For this review, use the dimensioned drawing (mm, ordinates from the lowest corner) and the shaded views. A direction names the side the tool comes from. Coordinates: 2 decimals unless noted, no trailing zeros. Write each loop counter-clockwise with the first axis right and the second up, starting at its lowest first coordinate (ties: lowest second). Pieces come first, ordered by that corner, then holes. Notation, with made-up numbers: (30, -12.75) - (88, -12.75) arc R30 cw to (88, 18.25) - close; hole circle Ø3 at (86.25, 82). An arc over 180 degrees is marked (long way). One line per item, written item: value.
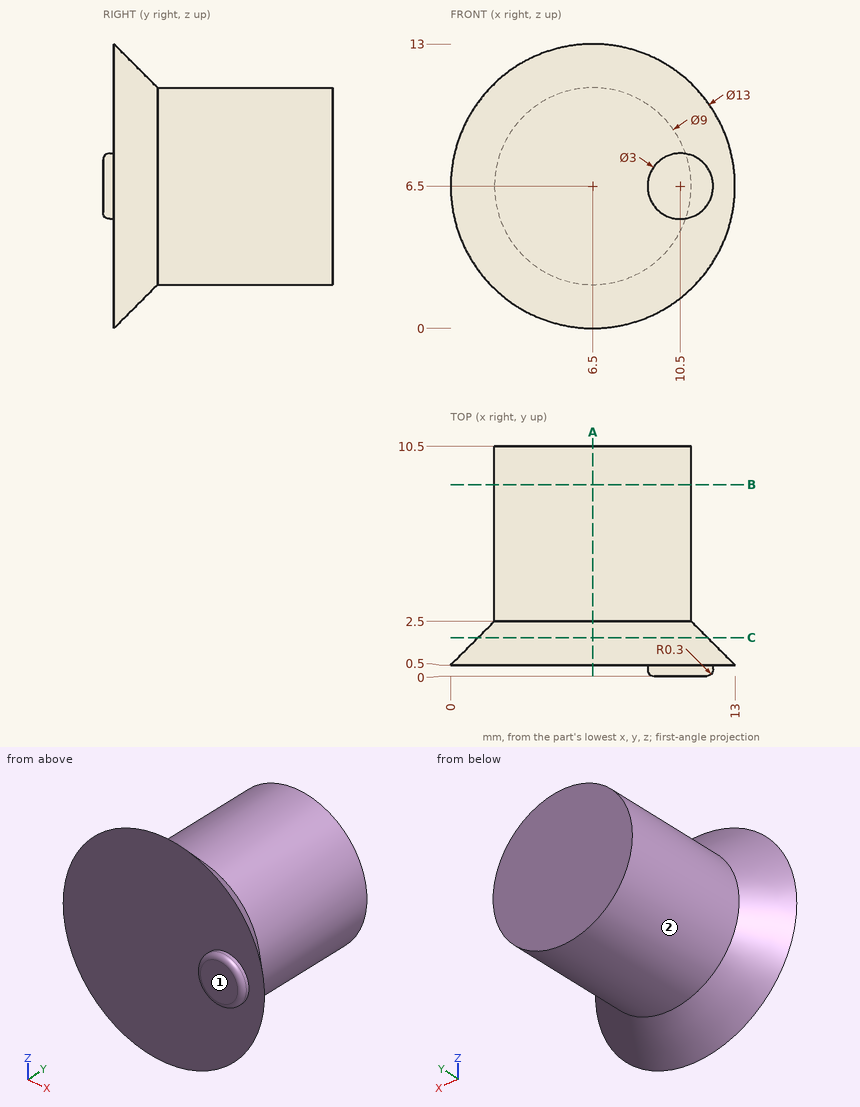
1. Consider section C-C, the plane y = 1.75. Write out the cut boundary in (x, z).
Answer block:
outline: circle Ø10.5 at (6.5, 6.5)
2. Wall thickness on line 1 along Y through (x, z) = (7.5, 10); line 2 along Y through (x, z) = (7, 12.25); line 3 along Z through (x, y) = (7, 8): over which ranges is each line inside the solid? List them lowest first.
Answer block:
line 1: y = 0.5 to 10.5
line 2: y = 0.5 to 1.23
line 3: z = 2.03 to 10.97
3. Consider section B-B, the plane y = 8.75. Write out the cut boundary in (x, z).
Answer block:
outline: circle Ø9 at (6.5, 6.5)
4. Insertion check: pin 1 Ø3 at (x, z) = (3, 10.5) entering from -Y; pin 2 Ø1 at (x, z) = (8, 2) entering from +Y; pin 3 Ø4 at (y, z) = (9.5, 2.5) entering from -X; pin 4 Ø4 at (x, y) = (6, 3) entering from +Z. Each pin has a flat end and moves straight along its axis. Give the tip position at first contact, or say it passes through.
Answer block:
pin 1: stops at y = 0.5
pin 2: stops at y = 10.5
pin 3: stops at x = 2.47
pin 4: stops at z = 12.48
5. For the marked faces 1 and 2, list the 3-axis set-ups (+Z, -Z, +X, -X, +Y, -Y) from which the entire face can be reached by the end or side of a thin tool; tool diameter is ignored.
Answer block:
face 1: +Z, -Z, +X, -X, -Y
face 2: +Y
6. Consider section A-A, the plane x = 6.5. Write out the cut boundary in (y, z).
Answer block:
outline: (0.5, 0) - (2.5, 2) - (10.5, 2) - (10.5, 11) - (2.5, 11) - (0.5, 13) - close
